from build123d import *

# Parameters (mm, degrees)
SKETCH1_R            = 11.1125
BOSS_EXTRUDE1_DEPTH  = 9.525
CHAMFER1_SIZE        = 0.79375
BOSS_EXTRUDE30_DEPTH = 2.38125


with BuildPart() as part:
    # Sketch1 → Boss-Extrude1 (new body)
    with BuildSketch(Plane(origin=(0, 0, 0), x_dir=(1, 0, 0), z_dir=(0, 1, 0))):
        with Locations(Location((0, 0, 0), (0, 0, 90))):
            Circle(SKETCH1_R)
    extrude(amount=BOSS_EXTRUDE1_DEPTH)

    # Chamfer1
    chamfer1_edges = [part.edges().sort_by_distance(p)[0] for p in [
        (0, 9.525, 11.1125),
    ]]
    chamfer(chamfer1_edges, length=CHAMFER1_SIZE)

    # Sketch2 → Boss-Extrude30 (add, symmetric)
    with BuildSketch(Plane.XY):
        with BuildLine():
            Line((11.049, 8.73125), (11.049, 11.90625))
            Line((11.049, 11.90625), (5.49275, 17.4625))
            Line((5.49275, 17.4625), (-16.73225, 17.4625))
            ThreePointArc((-16.73225, 17.4625), (-22.2885, 11.90625), (-16.73225, 6.35))
            Line((-16.73225, 6.35), (-11.176, 6.35))
            Line((-11.176, 6.35), (-11.176, 8.73125))
            Line((-11.176, 8.73125), (-10.38225, 9.525))
            Line((-10.38225, 9.525), (10.25525, 9.525))
            Line((10.25525, 9.525), (11.049, 8.73125))
        make_face()
    extrude(amount=BOSS_EXTRUDE30_DEPTH, both=True)


solid = part.part
Read the model definition and answer for the solid it produces. Units are mm, in the model's axes. A direction names the side the tool comes from. Coordinates: 2 decimals unless noted, no trailing zeros. Loops run counter-clockwise (first coordinate to the right, second up) from the corner with the lowest first, then second, coordinate; pieces in that order, holes last.
Q1. The part is cut by section B-B on x = 0. Write down the section's boundary in (y, z) (1 decimal), and give its area (3 significant figures).
Q2. Consider probe 1 along Y at (x, z) = (8, -3) (3 decimals); probe 2 along Z at (x, y) = (-4.5, 14.25); probe 3 along Y at (x, z) = (-13.5, -1.25). Determine where each line is inside the solid, lowest interval first.
Q3. The part is cut by section C-C on y = 7.5. Write down the section's boundary in (x, z) (1 decimal).
Q4. Each of these flat-tipped pins is pushed along its axis until it touches: pin 1 Ø1 at (y, z) = (10.5, 0.5) entering from +X; pin 2 Ø2.5 at (x, z) = (-14.5, -0.5) entering from -Y; pin 3 Ø3 at (x, y) = (-15.5, 15) entering from +Z; pin 4 Ø1.5 at (y, z) = (15.5, 4.5) entering from -X. Where does it stop, or does it pass through?
Q5. Which of the six approach directions +Z, -Z, +X, -X, +Y, -Y give full straight-line access (tool end or side, diameter ignored) to faces 1 (the face through (0, 9.525, 6)), 2 (the face through (-14, 6.35, 0)), 3 (the face through (0, 9.525, -5))?
Results below:
1. outline: (0, -11.1) - (8.7, -11.1) - (9.5, -10.3) - (9.5, -2.4) - (17.5, -2.4) - (17.5, 2.4) - (9.5, 2.4) - (9.5, 10.3) - (8.7, 11.1) - (0, 11.1) - close
1. area: 249 mm2
2. probe 1: y = 0 to 9.525
2. probe 2: z = -2.38 to 2.38
2. probe 3: y = 6.35 to 17.46
3. outline: (-20.1, -2.4) - (-11.2, -2.4) - (-11.2, 2.4) - (-20.1, 2.4) - close; circle Ø22.2 at (0, 0)
4. pin 1: stops at x = 11.05
4. pin 2: stops at y = 6.35
4. pin 3: stops at z = 2.38
4. pin 4: passes through
5. face 1: +Z, +X, -X, +Y
5. face 2: +Z, -Z, -X, -Y
5. face 3: -Z, +X, -X, +Y
